from build123d import *

# Parameters (mm, degrees)
BOSS_EXTRUDE1_DEPTH      = 10
BOSS_EXTRUDE1_DEPTH_BACK = 10
SKETCH1_R                = 15
SKETCH2_R                = 20.25
CUT_EXTRUDE1_DEPTH       = 5


with BuildPart() as part:
    # Sketch1 → Boss-Extrude1 (new, two sides: drawn at the far end of the back side and taken through both)
    with BuildSketch(Plane.XY.offset(-BOSS_EXTRUDE1_DEPTH_BACK)):
        with BuildLine():
            Line((-1.2, 30), (1.2, 30))
            Line((1.2, 30), (3, 24.819347292))
            ThreePointArc((3, 24.819347292), (3.910861626, 24.692208515), (4.816430554, 24.531652955))
            Line((4.816430554, 24.531652955), (8.129242012, 28.902515882))
            Line((8.129242012, 28.902515882), (10.411777651, 28.160875096))
            Line((10.411777651, 28.160875096), (10.522769651, 22.677550989))
            ThreePointArc((10.522769651, 22.677550989), (11.349762493, 22.275163105), (12.161395327, 21.842629505))
            Line((12.161395327, 21.842629505), (16.662737176, 24.975852134))
            Line((16.662737176, 24.975852134), (18.604377962, 23.565167528))
            Line((18.604377962, 23.565167528), (17.015497293, 18.315917992))
            ThreePointArc((17.015497293, 18.315917992), (17.67766953, 17.67766953), (18.315917992, 17.015497293))
            Line((18.315917992, 17.015497293), (23.565167528, 18.604377962))
            Line((23.565167528, 18.604377962), (24.975852134, 16.662737176))
            Line((24.975852134, 16.662737176), (21.842629505, 12.161395327))
            ThreePointArc((21.842629505, 12.161395327), (22.275163105, 11.349762493), (22.677550989, 10.522769651))
            Line((22.677550989, 10.522769651), (28.160875096, 10.411777651))
            Line((28.160875096, 10.411777651), (28.902515882, 8.129242012))
            Line((28.902515882, 8.129242012), (24.531652955, 4.816430554))
            ThreePointArc((24.531652955, 4.816430554), (24.692208515, 3.910861626), (24.819347292, 3))
            Line((24.819347292, 3), (30, 1.2))
            Line((30, 1.2), (30, -1.2))
            Line((30, -1.2), (24.819347292, -3))
            ThreePointArc((24.819347292, -3), (24.692208515, -3.910861626), (24.531652955, -4.816430554))
            Line((24.531652955, -4.816430554), (28.902515882, -8.129242012))
            Line((28.902515882, -8.129242012), (28.160875096, -10.411777651))
            Line((28.160875096, -10.411777651), (22.677550989, -10.522769651))
            ThreePointArc((22.677550989, -10.522769651), (22.275163105, -11.349762493), (21.842629505, -12.161395327))
            Line((21.842629505, -12.161395327), (24.975852134, -16.662737176))
            Line((24.975852134, -16.662737176), (23.565167528, -18.604377962))
            Line((23.565167528, -18.604377962), (18.315917992, -17.015497293))
            ThreePointArc((18.315917992, -17.015497293), (17.67766953, -17.67766953), (17.015497293, -18.315917992))
            Line((17.015497293, -18.315917992), (18.604377962, -23.565167528))
            Line((18.604377962, -23.565167528), (16.662737176, -24.975852134))
            Line((16.662737176, -24.975852134), (12.161395327, -21.842629505))
            ThreePointArc((12.161395327, -21.842629505), (11.349762493, -22.275163105), (10.522769651, -22.677550989))
            Line((10.522769651, -22.677550989), (10.411777651, -28.160875096))
            Line((10.411777651, -28.160875096), (8.129242012, -28.902515882))
            Line((8.129242012, -28.902515882), (4.816430554, -24.531652955))
            ThreePointArc((4.816430554, -24.531652955), (3.910861626, -24.692208515), (3, -24.819347292))
            Line((3, -24.819347292), (1.2, -30))
            Line((1.2, -30), (-1.2, -30))
            Line((-1.2, -30), (-3, -24.819347292))
            ThreePointArc((-3, -24.819347292), (-3.910861626, -24.692208515), (-4.816430554, -24.531652955))
            Line((-4.816430554, -24.531652955), (-8.129242012, -28.902515882))
            Line((-8.129242012, -28.902515882), (-10.411777651, -28.160875096))
            Line((-10.411777651, -28.160875096), (-10.522769651, -22.677550989))
            ThreePointArc((-10.522769651, -22.677550989), (-11.349762493, -22.275163105), (-12.161395327, -21.842629505))
            Line((-12.161395327, -21.842629505), (-16.662737176, -24.975852134))
            Line((-16.662737176, -24.975852134), (-18.604377962, -23.565167528))
            Line((-18.604377962, -23.565167528), (-17.015497293, -18.315917992))
            ThreePointArc((-17.015497293, -18.315917992), (-17.67766953, -17.67766953), (-18.315917992, -17.015497293))
            Line((-18.315917992, -17.015497293), (-23.565167528, -18.604377962))
            Line((-23.565167528, -18.604377962), (-24.975852134, -16.662737176))
            Line((-24.975852134, -16.662737176), (-21.842629505, -12.161395327))
            ThreePointArc((-21.842629505, -12.161395327), (-22.275163105, -11.349762493), (-22.677550989, -10.522769651))
            Line((-22.677550989, -10.522769651), (-28.160875096, -10.411777651))
            Line((-28.160875096, -10.411777651), (-28.902515882, -8.129242012))
            Line((-28.902515882, -8.129242012), (-24.531652955, -4.816430554))
            ThreePointArc((-24.531652955, -4.816430554), (-24.692208515, -3.910861626), (-24.819347292, -3))
            Line((-24.819347292, -3), (-30, -1.2))
            Line((-30, -1.2), (-30, 1.2))
            Line((-30, 1.2), (-24.819347292, 3))
            ThreePointArc((-24.819347292, 3), (-24.692208515, 3.910861626), (-24.531652955, 4.816430554))
            Line((-24.531652955, 4.816430554), (-28.902515882, 8.129242012))
            Line((-28.902515882, 8.129242012), (-28.160875096, 10.411777651))
            Line((-28.160875096, 10.411777651), (-22.677550989, 10.522769651))
            ThreePointArc((-22.677550989, 10.522769651), (-22.275163105, 11.349762493), (-21.842629505, 12.161395327))
            Line((-21.842629505, 12.161395327), (-24.975852134, 16.662737176))
            Line((-24.975852134, 16.662737176), (-23.565167528, 18.604377962))
            Line((-23.565167528, 18.604377962), (-18.315917992, 17.015497293))
            ThreePointArc((-18.315917992, 17.015497293), (-17.67766953, 17.67766953), (-17.015497293, 18.315917992))
            Line((-17.015497293, 18.315917992), (-18.604377962, 23.565167528))
            Line((-18.604377962, 23.565167528), (-16.662737176, 24.975852134))
            Line((-16.662737176, 24.975852134), (-12.161395327, 21.842629505))
            ThreePointArc((-12.161395327, 21.842629505), (-11.349762493, 22.275163105), (-10.522769651, 22.677550989))
            Line((-10.522769651, 22.677550989), (-10.411777651, 28.160875096))
            Line((-10.411777651, 28.160875096), (-8.129242012, 28.902515882))
            Line((-8.129242012, 28.902515882), (-4.816430554, 24.531652955))
            ThreePointArc((-4.816430554, 24.531652955), (-3.910861626, 24.692208515), (-3, 24.819347292))
            Line((-3, 24.819347292), (-1.2, 30))
        make_face()
        Circle(SKETCH1_R, mode=Mode.SUBTRACT)
    extrude(amount=BOSS_EXTRUDE1_DEPTH + BOSS_EXTRUDE1_DEPTH_BACK)

    # Sketch2 → Cut-Extrude1 (cut)
    with BuildSketch(Plane.XY.offset(10)):
        Circle(SKETCH2_R)
    cut_extrude1 = extrude(amount=-CUT_EXTRUDE1_DEPTH, mode=Mode.SUBTRACT)

    # Mirror1: Cut-Extrude1 across plane
    add(cut_extrude1.mirror(Plane.XY), mode=Mode.SUBTRACT)


solid = part.part
Could you check a few things on this model? Use its own coordinates, in mm. A direction names the side the tool comes from. Give positions to 0.01 mm unless a question says otherwise; leave off trailing zeros. Order: outer loops, then holes, each group sorted by start corner. A loop starts at its lowest first (then second) coordinate and runs counter-clockwise, first axis right, second up.
1. Will these pins go through, and if not, where does the flat tip stop? P1, Ø20, axis at x = -5, y = -2.5, coming from the -Z side; P2, Ø6, axis at x = -13, z = -6.5, coming from the -Y side; P3, Ø8, axis at x = 19.5, z = -7, coming from the -Y side.
2. I need wall thicknesses on L1, parallel to Y at x = 0, z = 6.7; L2, parallel to Y at x = -22, z = -1.5; L3, parallel to Y at x = 0, z = 2. Which ranges of each line are inside material? Lowest first, please.
3. Suppose I cut it at A-A (y = 0). List the corners of the cut face in (x, z) for me, plus the area to 3 significant figures.
4. For faces 4 (the cylindrical face through (11, 17, -8)), 5 (the flat face through (-2.087, -27.446, -0.14)), 6 (the flat face through (-26.75, -6.5, -0.14)), 7 (the flat face through (26.75, 6.5, -0.14)), which set-ups out of +Z, -Z, +X, -X, +Y, -Y let a thin tool reach every point of the face, with its end or its side?
5. We'd pull the mould along Y, two halves only. Please class faces 1 (the flat face through (24.28, -17.62, -0.14)), 2 (the flat face through (23.4, -14.4, -0.1)), 3 (the cylindrical face through (11.3, 22.3, -0.1)): pulls with the +Y half, pulls with the -Y half, needs draft (parallel to the pull), parting line crosses it, or undercut.
Solved:
1. P1: stops at z = -5
1. P2: stops at y = -28.29
1. P3: stops at y = -24.98
2. L1: y = -30 to -20.25, 20.25 to 30
2. L2: y = -18.13 to -12.39, -11.87 to 11.87, 12.39 to 18.13
2. L3: y = -30 to -15, 15 to 30
3. outline: (-30, -10) - (-20.25, -10) - (-20.25, -5) - (-15, -5) - (-15, 5) - (-20.25, 5) - (-20.25, 10) - (-30, 10) - close; (15, -5) - (20.25, -5) - (20.25, -10) - (30, -10) - (30, 10) - (20.25, 10) - (20.25, 5) - (15, 5) - close
3. area: 495 mm2
4. face 4: -Z
4. face 5: +Z, -Z, -Y
4. face 6: +Z, -Z, -X
4. face 7: +Z, -Z, +X
5. face 1: pulls with the -Y half
5. face 2: undercut
5. face 3: pulls with the +Y half
